Design review of the part built by this model. Coordinates are the model's own, in mm. Give positions to 0.01 mm unless a question says otherwise; leave off trailing zeros. Order: outer loops, then holes, each group sorted by start corner. A loop starts at its lowest first (then second) coordinate and runs counter-clockwise, first axis right, second up.
```python
from build123d import *

# Parameters (mm, degrees)
SKETCH1_R           = 0.5
SKETCH1_W           = 4.6
SKETCH1_H           = 0.5
BOSS_EXTRUDE1_DEPTH = 0.35


with BuildPart() as part:
    # Sketch1 → Boss-Extrude1 (new body)
    with BuildSketch(Plane(origin=(0, 0, 0), x_dir=(0, 0, -1), z_dir=(1, 0, 0))):
        with BuildLine():
            Line((16.515570225, 0.949375895), (0, 0.65))
            ThreePointArc((0, 0.65), (-0.65, 0), (0, -0.65))
            Line((0, -0.65), (16.515570225, -0.949375895))
            Line((16.515570225, -0.949375895), (16.55, -0.95))
            ThreePointArc((16.55, -0.95), (17.5, 0), (16.55, 0.95))
            Line((16.55, 0.95), (16.515570225, 0.949375895))
        make_face()
        Circle(SKETCH1_R, mode=Mode.SUBTRACT)
        with Locations((4.32, 0)):
            Rectangle(SKETCH1_W, SKETCH1_H, mode=Mode.SUBTRACT)
        with Locations((16.55, 0)):
            Circle(SKETCH1_R, mode=Mode.SUBTRACT)
    extrude(amount=BOSS_EXTRUDE1_DEPTH)


solid = part.part
```
1. Take a section at A-A (x = 0.2). State the section outline as (y, z) points, then the cut area to 3 significant figures.
Recorded:
outline: (-0.95, -16.55) arc R0.95 ccw to (0.95, -16.55) - (0.65, 0) arc R0.65 ccw to (-0.65, 0) - close; hole circle Ø1 at (0, -16.55); hole circle Ø1 at (0, 0); hole (-0.25, -6.62) - (0.25, -6.62) - (0.25, -2.02) - (-0.25, -2.02) - close
area: 24.7 mm2
2. Take a section at B-B (y = 0). State the section outline as (x, z) points.
Recorded:
outline: (0, -17.5) - (0.35, -17.5) - (0.35, -17.05) - (0, -17.05) - close; (0, -16.05) - (0.35, -16.05) - (0.35, -6.62) - (0, -6.62) - close; (0, -2.02) - (0.35, -2.02) - (0.35, -0.5) - (0, -0.5) - close; (0, 0.5) - (0.35, 0.5) - (0.35, 0.65) - (0, 0.65) - close
3. Take a section at C-C (z = -3). State the section outline as (x, y) points.
Recorded:
outline: (0, -0.7) - (0.35, -0.7) - (0.35, -0.25) - (0, -0.25) - close; (0, 0.25) - (0.35, 0.25) - (0.35, 0.7) - (0, 0.7) - close
4. Take a section at D-D (z = -7.25). State the section outline as (x, y) points.
Recorded:
outline: (0, -0.78) - (0.35, -0.78) - (0.35, 0.78) - (0, 0.78) - close
5. For line 1 along Y through (x, z) = (0.2, -16.55); line 2 along Z through (x, y) = (0.05, -0.2); line 3 along Y through (x, z) = (0.25, -4.75), list the stretches that pass through material, from the lowest coordinate up.
Recorded:
line 1: y = -0.95 to -0.5, 0.5 to 0.95
line 2: z = -17.48 to -17.01, -16.09 to -6.62, -2.02 to -0.46, 0.46 to 0.62
line 3: y = -0.74 to -0.25, 0.25 to 0.74
6. Draft analysis for pull direction Z (two halves, no side actions). For faces 1 (the face through (0, 0, -10)), 2 (the face through (0.17, -0.02, -17.5)), 3 (the face through (0.173, -0.488, 0.108)), state which applies: pulls with the +Z half, pulls with the -Z half, needs draft (parallel to the pull), parting line crosses it, or undercut.
Recorded:
face 1: needs draft
face 2: pulls with the -Z half
face 3: undercut
